Source: three-view drawing plus pictorial views. Frame: mm from the lowest corner of the part. A direction names the side the tool comes from. Coordinates: 2 decimals unless noted, no trailing zeros. Loops run counter-clockwise (first coordinate to the right, second up) from the corner with the lowest first, then second, coordinate; pieces in that order, holes last. Notation, with made-up numbers: (83, 83) - (96, 83) arc R26 cw to (96, 121) - close; hole circle Ø6 at (81, 46.5). An arc over 180 degrees is marked (long way). Use CSV: the item, a comma, the result in double quotes. Start each with the question number.
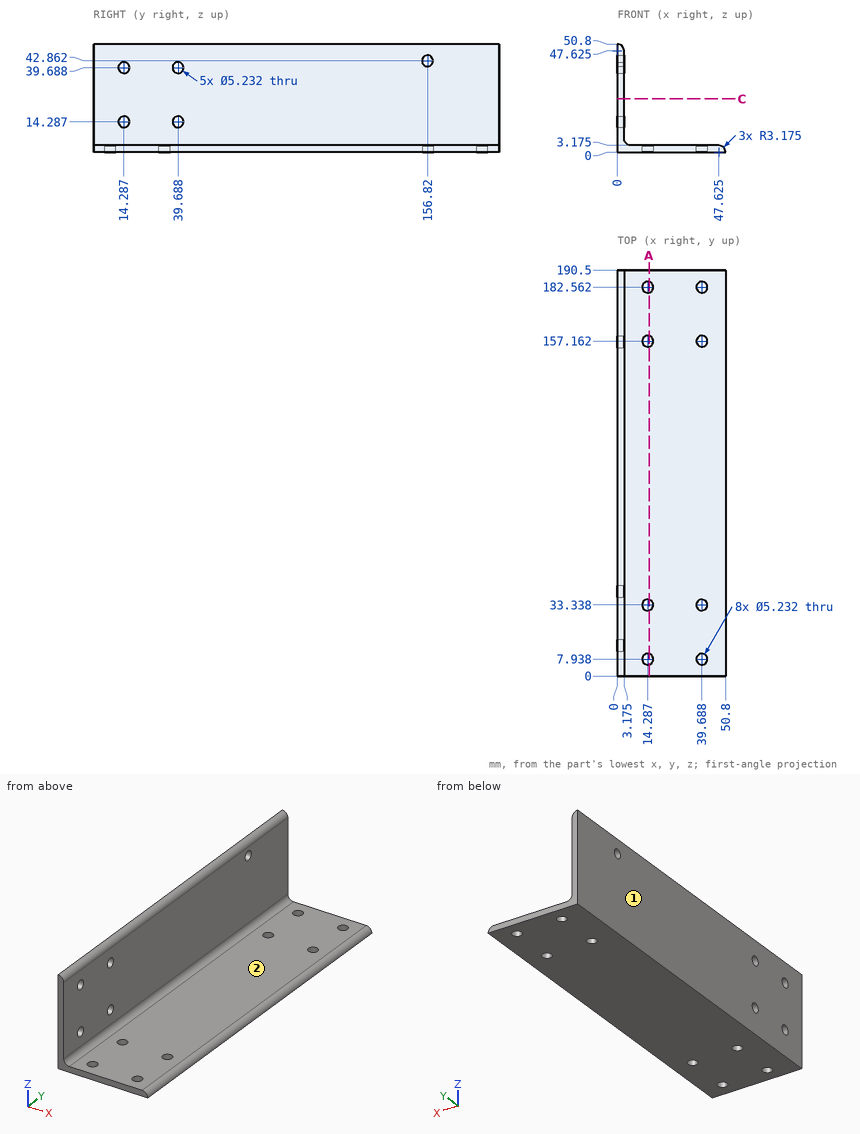
(1) Ray query, line 1 (X direction, y = 17, z = 14.5) (1 decimal); line 2 (Z direction, x = 5.5, y = 26.5). Return the intervals inside material, ascending. Write a range as [from, to].
(2) Reachability of the marked faces 1 and 2 from +Z, -Z, +X, -X, +Y, -Y: full face, straight path, thin tool, end or side. Return the list, or none.
(3) Pin query (flat end, axial travel): pin 1 Ø4 at (x, y) = (14.29, 33.34) entering from -Z; pin 2 Ø12 at (x, y) = (12.5, 158) entering from +Z (1 decimal); pin 3 Ø2 at (y, z) = (35.5, 42) entering from +X (1 decimal). Return the tip coordinate at first contact, or that it passes through.
(4) Section A-A on x = 15. Output: boundary loops of the cut face in (y, z) (1 decimal), plus the area to 3 significant figures.
(5) Section C-C on z = 25. Output: boundary loops of the cut face in (x, y) (1 decimal).
Solution:
1,line 1,"x = [0, 3.2]"
1,line 2,"z = [0, 3.29]"
2,face 1,"+Z, -Z, -X, +Y, -Y"
2,face 2,"+Z, +X, +Y, -Y"
3,pin 1,"passes through"
3,pin 2,"stops at z = 3.2"
3,pin 3,"stops at x = 3.2"
4,outline,"(0, 0) - (5.4, 0) - (5.4, 3.2) - (0, 3.2) - close; (10.5, 0) - (30.8, 0) - (30.8, 3.2) - (10.5, 3.2) - close; (35.9, 0) - (154.6, 0) - (154.6, 3.2) - (35.9, 3.2) - close; (159.7, 0) - (180, 0) - (180, 3.2) - (159.7, 3.2) - close; (185.1, 0) - (190.5, 0) - (190.5, 3.2) - (185.1, 3.2) - close"
4,area,"541 mm²"
5,outline,"(0, 0) - (3.2, 0) - (3.2, 190.5) - (0, 190.5) - close"
